```python
from build123d import *

# Parameters (mm, degrees)
SKETCH1_W           = 12.7
SKETCH1_H           = 139.7
SKETCH1_R           = 3.1496
SKETCH1_R_2         = 1.27
SKETCH1_R_3         = 2.54
BOSS_EXTRUDE1_DEPTH = 1.5875


with BuildPart() as part:
    # Sketch1 → Boss-Extrude1 (new body)
    with BuildSketch(Plane.XY):
        Rectangle(SKETCH1_W, SKETCH1_H)
        Circle(SKETCH1_R, mode=Mode.SUBTRACT)
        with Locations((0, 63.5)):
            Circle(SKETCH1_R_2, mode=Mode.SUBTRACT)
        with Locations(Location((0, -63.5, 0), (0, 0, 180))):
            Circle(SKETCH1_R_3, mode=Mode.SUBTRACT)
    extrude(amount=BOSS_EXTRUDE1_DEPTH)


solid = part.part
```
The model under review builds one solid part; all positions refer to its coordinate system, in mm. Round coordinates to 2 decimals unless told otherwise and drop trailing zeros. Loops run counter-clockwise (first coordinate to the right, second up) from the corner with the lowest first, then second, coordinate; pieces in that order, holes last. Notation, with made-up numbers: (64, 22.5) -> (80, 22.5) arc R18 ccw to (80, 31.5) -> close; hole circle Ø9 at (86.5, 46). An arc over 180 degrees is marked (long way). Answer in a Markdown table with one row per item.
1) For pin 1 Ø4.5 at (x, y) = (0, -63.5) entering from -Z; pin 2 Ø3 at (x, y) = (0, 63.5) entering from +Z, all flat-tipped, find the tip position at first contact; note any pin that passes through.
Taken from the geometry:
| item | result |
|---|---|
| pin 1 | passes through |
| pin 2 | stops at z = 1.59 |
2) Wall thickness on line 1 along Y through (x, z) = (0, 0.65); line 2 along Y through (x, z) = (-2, 1.3); line 3 along Y through (x, z) = (-1.5, 0.9): over which ranges is each line inside the solid? List them lowest first.
Taken from the geometry:
| item | result |
|---|---|
| line 1 | y = -69.85 to -66.04, -60.96 to -3.15, 3.15 to 62.23, 64.77 to 69.85 |
| line 2 | y = -69.85 to -65.07, -61.93 to -2.43, 2.43 to 69.85 |
| line 3 | y = -69.85 to -65.55, -61.45 to -2.77, 2.77 to 69.85 |
3) Consider section B-B, the plane x = 0. Write out the cut boundary in (y, z).
Taken from the geometry:
| item | result |
|---|---|
| outline | (-69.85, 0) -> (-66.04, 0) -> (-66.04, 1.59) -> (-69.85, 1.59) -> close; (-60.96, 0) -> (-3.15, 0) -> (-3.15, 1.59) -> (-60.96, 1.59) -> close; (3.15, 0) -> (62.23, 0) -> (62.23, 1.59) -> (3.15, 1.59) -> close; (64.77, 0) -> (69.85, 0) -> (69.85, 1.59) -> (64.77, 1.59) -> close |
4) Consider section D-D, the plane y = -63.5. Write out the cut boundary in (x, z).
Taken from the geometry:
| item | result |
|---|---|
| outline | (-6.35, 0) -> (-2.54, 0) -> (-2.54, 1.59) -> (-6.35, 1.59) -> close; (2.54, 0) -> (6.35, 0) -> (6.35, 1.59) -> (2.54, 1.59) -> close |
5) Consider section C-C, the plane z = 0.65. Write out the cut boundary in (x, y).
Taken from the geometry:
| item | result |
|---|---|
| outline | (-6.35, -69.85) -> (6.35, -69.85) -> (6.35, 69.85) -> (-6.35, 69.85) -> close; hole circle Ø6.3 at (0, 0); hole circle Ø5.08 at (0, -63.5); hole circle Ø2.54 at (0, 63.5) |
6) Consider section A-A, the plane y = 63.5. Write out the cut boundary in (x, z).
Taken from the geometry:
| item | result |
|---|---|
| outline | (-6.35, 0) -> (-1.27, 0) -> (-1.27, 1.59) -> (-6.35, 1.59) -> close; (1.27, 0) -> (6.35, 0) -> (6.35, 1.59) -> (1.27, 1.59) -> close |
7) Draft analysis for pull direction X (two halves, no side actions). For faces 1 (the flat face through (4, 1, 1.588)), 2 (the cylindrical face through (0.55, -61.02, 0.78)), state which applies: pulls with the +X half, pulls with the -X half, needs draft (parallel to the pull), parting line crosses it, or undercut.
Taken from the geometry:
| item | result |
|---|---|
| face 1 | needs draft |
| face 2 | undercut |
